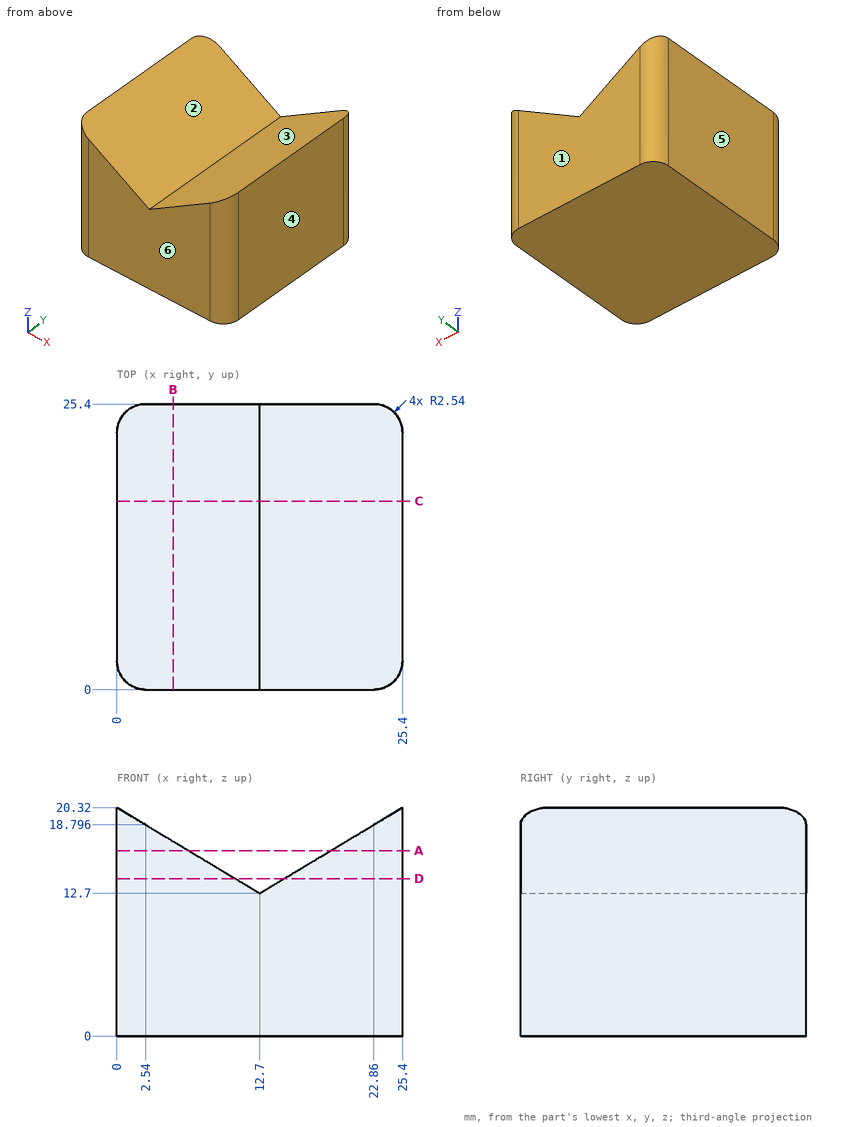
Job drawing, mm, ordinate dimensions from the low corner. One solid piece. A direction names the side the tool comes from. Give positions to 0.01 mm unless a question says otherwise; leave off trailing zeros. Write each loop counter-clockwise with the first axis right and the second up, starting at its lowest first coordinate (ties: lowest second). Pieces come first, ordered by that corner, then holes. Notation, with made-up numbers: (-22, 20.25) - (12, 20.25) arc R8 ccw to (12, 35.25) - close; hole circle Ø7 at (78, -16). An arc over 180 degrees is marked (long way). Answer as CSV lines item,"result".
1. Band-saw the part on D-D (z = 14). Write the cut outline in (x, y).
Responses:
outline,"(0, 2.54) arc R2.54 ccw to (2.54, 0) - (10.53, 0) - (10.53, 25.4) - (2.54, 25.4) arc R2.54 ccw to (0, 22.86) - close; (14.87, 0) - (22.86, 0) arc R2.54 ccw to (25.4, 2.54) - (25.4, 22.86) arc R2.54 ccw to (22.86, 25.4) - (14.87, 25.4) - close"
2. Band-saw the part on C-C (y = 16.75). Write the cut outline in (x, z).
Responses:
outline,"(0, 0) - (25.4, 0) - (25.4, 20.32) - (12.7, 12.7) - (0, 20.32) - close"
3. Two-plate mould, pull along X, no slides. Class the marked faces 3, 4, 5 and 6: +X half, -X half, draft (parallel to the pull), parting line (faces both ways), or undercut.
Responses:
face 3,"undercut"
face 4,"+X half"
face 5,"-X half"
face 6,"draft"
4. Band-saw the part on B-B (x = 5). Write the cut outline in (y, z).
Responses:
outline,"(0, 0) - (25.4, 0) - (25.4, 17.32) - (0, 17.32) - close"
5. 3-axis set-ups, long thin cutter, end or side, ignore diameter. For the marked faces 1 and 2: which of +Z, -Z, +X, -X, +Y, -Y reach the whole face in a straight line?
Responses:
face 1,"+Z, -Z, +X, -X, +Y"
face 2,"+Z, +Y, -Y"
6. Drill centre lines: L1, parallel to X at y = 6.5, z = 14.5; L2, parallel to X at y = 6.25, z = 12.75; L3, parallel to Z at x = 19.5, y = 12.25. Where is each one in solid material? Low to high. Write a range as [from, to].
Responses:
L1,"x = [0, 9.7], [15.7, 25.4]"
L2,"x = [0, 12.62], [12.78, 25.4]"
L3,"z = [0, 16.78]"
7. Pin check, flat tip, straight feed: pin 1 (8 mm diameter, centred on x = 19, y = 22.5, fed in from +Z). Stop position of the tip, or through.
Responses:
pin 1,"stops at z = 18.88"
8. Band-saw the part on A-A (z = 16.5). Write the cut outline in (x, y).
Responses:
outline,"(0, 2.54) arc R2.54 ccw to (2.54, 0) - (6.37, 0) - (6.37, 25.4) - (2.54, 25.4) arc R2.54 ccw to (0, 22.86) - close; (19.03, 0) - (22.86, 0) arc R2.54 ccw to (25.4, 2.54) - (25.4, 22.86) arc R2.54 ccw to (22.86, 25.4) - (19.03, 25.4) - close"
